```python
from build123d import *

# Parameters (mm, degrees)
SKETCH1_W           = 1.2
SKETCH1_H           = 7.6
SKETCH1_W_2         = 19
SKETCH1_H_2         = 1.2
BOSS_EXTRUDE1_DEPTH = 299
SKETCH3_R           = 4.05
CUT_EXTRUDE2_DEPTH  = 370
CUT_EXTRUDE4_DEPTH  = 370


with BuildPart() as part:
    # Sketch1 → Boss-Extrude1 (new body)
    with BuildSketch(Plane.XY):
        Rectangle(SKETCH1_W, SKETCH1_H)
        with Locations((0, -4.4)):
            Rectangle(SKETCH1_W_2, SKETCH1_H_2)
        with Locations((0, 4.4)):
            Rectangle(SKETCH1_W_2, SKETCH1_H_2)
    extrude(amount=BOSS_EXTRUDE1_DEPTH)

    # Sketch3 → Cut-Extrude2 (cut)
    with BuildSketch(Plane(origin=(0, 5, 0), x_dir=(1, 0, 0), z_dir=(0, 1, 0))):
        with BuildLine():
            Line((-9.5, 0), (-9.5, -9.5))
            ThreePointArc((-9.5, -9.5), (-6.717514436, -2.782485594), (-4.2e-08, 0))
            Line((-4.2e-08, 0), (-9.5, 0))
        make_face()
        with BuildLine():
            Line((9.5, 0), (-4.2e-08, 0))
            ThreePointArc((-4.2e-08, 0), (6.717514406, -2.782485564), (9.5, -9.5))
            Line((9.5, -9.5), (9.5, 0))
        make_face()
        with BuildLine():
            ThreePointArc((14.5, -9.5), (0, 5), (-14.5, -9.5))
            Line((-14.5, -9.5), (-9.5, -9.5))
            Line((-9.5, -9.5), (-9.5, 0))
            Line((-9.5, 0), (-4.2e-08, 0))
            Line((-4.2e-08, 0), (9.5, 0))
            Line((9.5, 0), (9.5, -9.5))
            Line((9.5, -9.5), (14.5, -9.5))
        make_face()
        with Locations((0, -9.5)):
            Circle(SKETCH3_R)
    cut_extrude2 = extrude(amount=-CUT_EXTRUDE2_DEPTH, mode=Mode.SUBTRACT)

    # Mirror1: Cut-Extrude2 across plane
    add(cut_extrude2.mirror(Plane.XY.offset(149.5)), mode=Mode.SUBTRACT)

    # Sketch6 → Cut-Extrude4 (cut)
    with BuildSketch(Plane.ZY.offset(0.6)):
        with BuildLine():
            Line((20, -3.8), (-1, -3.8))
            Line((-1, -3.8), (-1, 3.8))
            Line((-1, 3.8), (20, 3.8))
            Line((20, 3.8), (20, 3.464101615))
            ThreePointArc((20, 3.464101615), (20.122035527, 3.13677478), (20.428571429, 2.969229956))
            ThreePointArc((20.428571429, 2.969229956), (23, 0), (20.428571429, -2.969229956))
            ThreePointArc((20.428571429, -2.969229956), (20.122035527, -3.13677478), (20, -3.464101615))
            Line((20, -3.464101615), (20, -3.8))
        make_face()
    cut_extrude4 = extrude(amount=-CUT_EXTRUDE4_DEPTH, mode=Mode.SUBTRACT)

    # Mirror3: Cut-Extrude4 across plane
    add(cut_extrude4.mirror(Plane.XY.offset(149.5)), mode=Mode.SUBTRACT)


solid = part.part
```
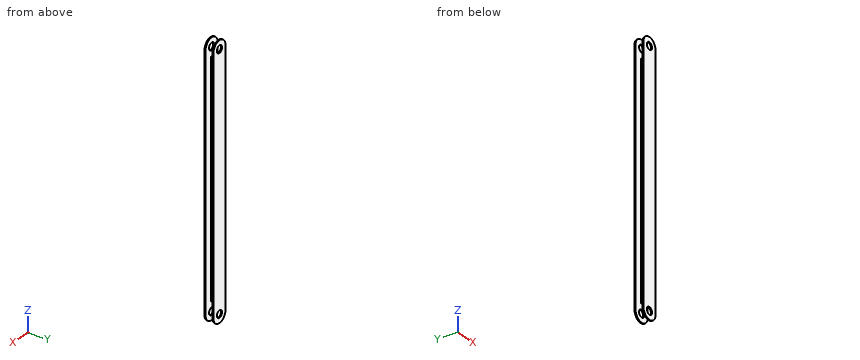
Here's how the part is built. I have some questions about the finished solid (model axes, mm). Give positions to 0.01 mm unless a question says otherwise; leave off trailing zeros. Loops run counter-clockwise (first coordinate to the right, second up) from the corner with the lowest first, then second, coordinate; pieces in that order, holes last. Notation, with made-up numbers: M 28.5,-37 L 61.5,-37 A19 ccw 61.5,-16 Z; hole C -10.5,46.25 d3. An arc over 180 degrees is marked long. Put each result on its own line as item: value. Start each with the question number.
(1) Will these pins go through, and if not, where does the flat tip stop? pin 1 Ø4 at (y, z) = (-1.5, 195) entering from +X; pin 2 Ø1.5 at (y, z) = (-3, 196.5) entering from -X.
(2) I need wall thicknesses on line 1 along Z through (x, y) = (0, -4.45); line 2 along Y through (x, z) = (8.75, 212); line 3 along X through (y, z) = (4.2, 9.5). Which ranges of each line are inside material? Lowest first, please. Write a range as [from, to].
(3) I want a section at A-A on z = 243. Please give me the cut outline in (x, y), then the cut area to 3 significant figures.
(4) I want a section at B-B on y = -0.75. Please give me the cut outline in (x, z), then the cut area to 3 significant figures.
Answer block:
1. pin 1: x = 0.6
1. pin 2: x = -0.6
2. line 1: [0, 5.45], [13.55, 285.45], [293.55, 299]
2. line 2: [-5, -3.8], [3.8, 5]
2. line 3: [-9.5, -4.05], [4.05, 9.5]
3. outline: M -9.5,-5 L 9.5,-5 L 9.5,-3.8 L 0.6,-3.8 L 0.6,3.8 L 9.5,3.8 L 9.5,5 L -9.5,5 L -9.5,3.8 L -0.6,3.8 L -0.6,-3.8 L -9.5,-3.8 Z
3. area: 54.7 mm^2
4. outline: M -0.6,22.9 L 0.6,22.9 L 0.6,276.1 L -0.6,276.1 Z
4. area: 304 mm^2
